The listing builds one solid part. Answer for the finished solid, in the listing's coordinates (mm). Face numbers are marked on the shaded views. A direction names the side the tool comes from. Coordinates: 2 decimals unless noted, no trailing zeros. Order: outer loops, then holes, each group sorted by start corner. A loop starts at its lowest first (then second) coordinate and runs counter-clockwise, first axis right, second up. Notation, with made-up numbers: (58, -25) - (62, -25) arc R23 cw to (62, -15) - close; hole circle Ø10 at (-26.5, -22.5). An arc over 180 degrees is marked (long way). Use a Markdown table: item, result. Add a question column.
Item 1: The part is cut by section A-A, the plane y = 28.5. Give the vertices of the cut face in (x, z).
Item 2: The part is cut by section B-B, the plane y = 40. Give the vertices of the cut face in (x, z).
Item 3: For the marked faces 4 and 5, determine the directions among +Z, -Z, +X, -X, +Y, -Y from which every point of the face is accessible in a straight line to the end or side of a thin tool.
Item 4: Find the intervals of material crossed by line 1 along X through (y, z) = (26.5, 0); line 2 along Y through (x, z) = (4.25, 8), in increasing order.
Item 5: The part is cut by section C-C, the plane y = 48. Give the vertices of the cut face in (x, z).
Item 6: The mould has two halves that part along Z. Classify the marked faces 1, 2 and 3: released by +Z, released by -Z, zero draft, split by the parting line, or undercut.
Item 7: Flat-ended cylindrical pins translate along their axes: P1, Ø5, axis at y = 46, z = 5, coming from the -X side; P2, Ø5, axis at x = 6, z = 5.5, coming from the -Y side; P3, Ø10, axis at x = 4, y = 30.5, coming from the -Z side. Find the tip coordinate at first contact, or state that the pin passes through.
from build123d import *

# Parameters (mm, degrees)
FILETE1_R     = 2
CHANFRO1_SIZE = 0.5


with BuildPart() as part:
    # Esboço1 → Revolução1 (revolve)
    with BuildSketch(Plane.XY):
        Polygon((0, 61.836212625), (12.75, 61.836212625), (12.75, 57.836212625), (6.95, 57.836212625), (6.95, 44.436212625), (5, 44.436212625), (5, 20.436212625), (2, 20.436212625), (2, 29.436212625), (0, 30.686212625), align=None)
    revolve(axis=Axis((0, -52.719767442, 0), (0, 1, 0)))

    # Filete1
    filete1_edges = [part.edges().sort_by_distance(p)[0] for p in [
        (-12.75, 57.836212625, 0),
        (-12.75, 61.836212625, 0),
    ]]
    fillet(filete1_edges, radius=FILETE1_R - 0.0001)  # a hair under: the kernel refuses the full size

    # Chanfro1
    chanfro1_edges = [part.edges().sort_by_distance(p)[0] for p in [
        (-5, 20.436212625, 0),
    ]]
    chamfer(chanfro1_edges, length=CHANFRO1_SIZE)


solid = part.part
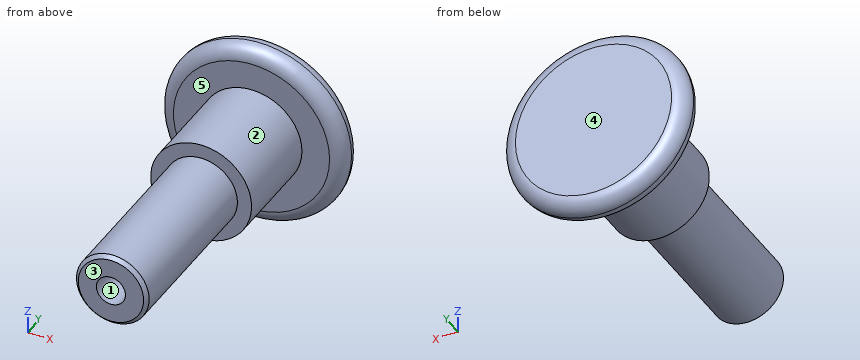
Solution:
| question | item | result |
|---|---|---|
| 1 | outline | circle Ø10 at (0, 0); hole circle Ø4 at (0, 0) |
| 2 | outline | circle Ø10 at (0, 0) |
| 3 | face 4 | +Z, -Z, +X, -X, +Y |
| 3 | face 5 | -Y |
| 4 | line 1 | x = -5 to -2, 2 to 5 |
| 4 | line 2 | y = 57.84 to 61.84 |
| 5 | outline | circle Ø13.9 at (0, 0) |
| 6 | face 1 | undercut |
| 6 | face 2 | split by the parting line |
| 6 | face 3 | zero draft |
| 7 | P1 | stops at x = -6.48 |
| 7 | P2 | stops at y = 44.44 |
| 7 | P3 | stops at z = -5 |
